Geometry: see drawing. Coordinates: mm, zero at the bounding-box minimum. A direction names the side the tool comes from. Coordinates: 2 decimals unless noted, no trailing zeros. Loops run counter-clockwise (first coordinate to the right, second up) from the corner with the lowest first, then second, coordinate; pieces in that order, holes last. Notation, with made-up numbers: (-14.75, 18.25) -> (21.25, 18.25) arc R30 cw to (21.25, 40.25) -> close; hole circle Ø4 at (-25, 15.25). An arc over 180 degrees is marked (long way). One line per item, written item: value. Start each with the question number.
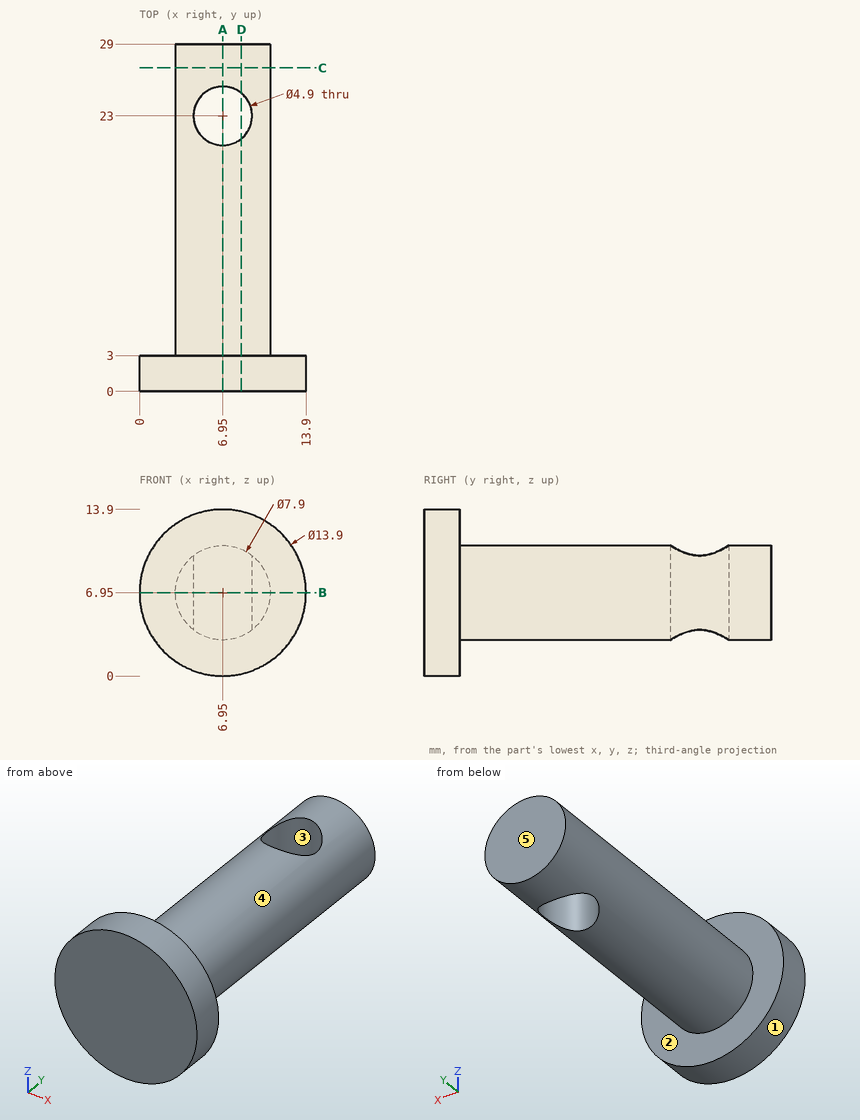
1. Draft query along X for the marked faces 3, 4 and 5. Return one class per face: released by +X, released by -X, zero draft, split by the parting line, or undercut.
2. Pin query (flat end, axial travel): pin 1 Ø8 at (y, z) = (15.5, 2) entering from +X; pin 2 Ø1.5 at (y, z) = (16.5, 12) entering from -X; pin 3 Ø6 at (x, y) = (7, 18.5) entering from +Z; pin 4 Ø8 at (y, z) = (22, 11) entering from -X. Return the tip coordinate at first contact, or that it passes through.
3. Set-up query: the marked faces 1 and 2. Return all of +Z, -Z, +X, -X, +Y, -Y with unobstructed straight access to the full face (end or side cutting, diameter ignored); none if empty.
4. Section A-A on x = 6.95. Return the cut outline in (y, z), plus the area to 3 significant figures.
5. Section D-D on x = 8.5. Return the cut outline in (y, z), plus the area to 3 significant figures.
6. Section C-C on y = 27. Return the cut outline in (x, z).
7. Section B-B on z = 6.95. Return the cut outline in (x, y), plus the area to 3 significant figures.
8. Line query: L1, parallel to Y at x = 6.95, z = 8; L2, parallel to X at y = 23, z = 7; L3, parallel to Y at x = 8.75, z = 0.5. Output: solid intervals per line, ascending. Write a range as [from, to].
Checks:
1. face 3: undercut
1. face 4: split by the parting line
1. face 5: zero draft
2. pin 1: x = 10.78
2. pin 2: through
2. pin 3: z = 10.9
2. pin 4: x = 3
3. face 1: +Y, -Y
3. face 2: +Y
4. outline: (0, 0) -> (3, 0) -> (3, 3) -> (20.55, 3) -> (20.55, 10.9) -> (3, 10.9) -> (3, 13.9) -> (0, 13.9) -> close; (25.45, 3) -> (29, 3) -> (29, 10.9) -> (25.45, 10.9) -> close
4. area: 208 mm²
5. outline: (0, 0.18) -> (3, 0.18) -> (3, 3.32) -> (21.1, 3.32) -> (21.1, 10.58) -> (3, 10.58) -> (3, 13.72) -> (0, 13.72) -> close; (24.9, 3.32) -> (29, 3.32) -> (29, 10.58) -> (24.9, 10.58) -> close
5. area: 202 mm²
6. outline: circle Ø7.9 at (6.95, 6.95)
7. outline: (0, 0) -> (13.9, 0) -> (13.9, 3) -> (10.9, 3) -> (10.9, 29) -> (3, 29) -> (3, 3) -> (0, 3) -> close; hole circle Ø4.9 at (6.95, 23)
7. area: 228 mm²
8. L1: [0, 20.55], [25.45, 29]
8. L2: [3, 4.5], [9.4, 10.9]
8. L3: [0, 3]
